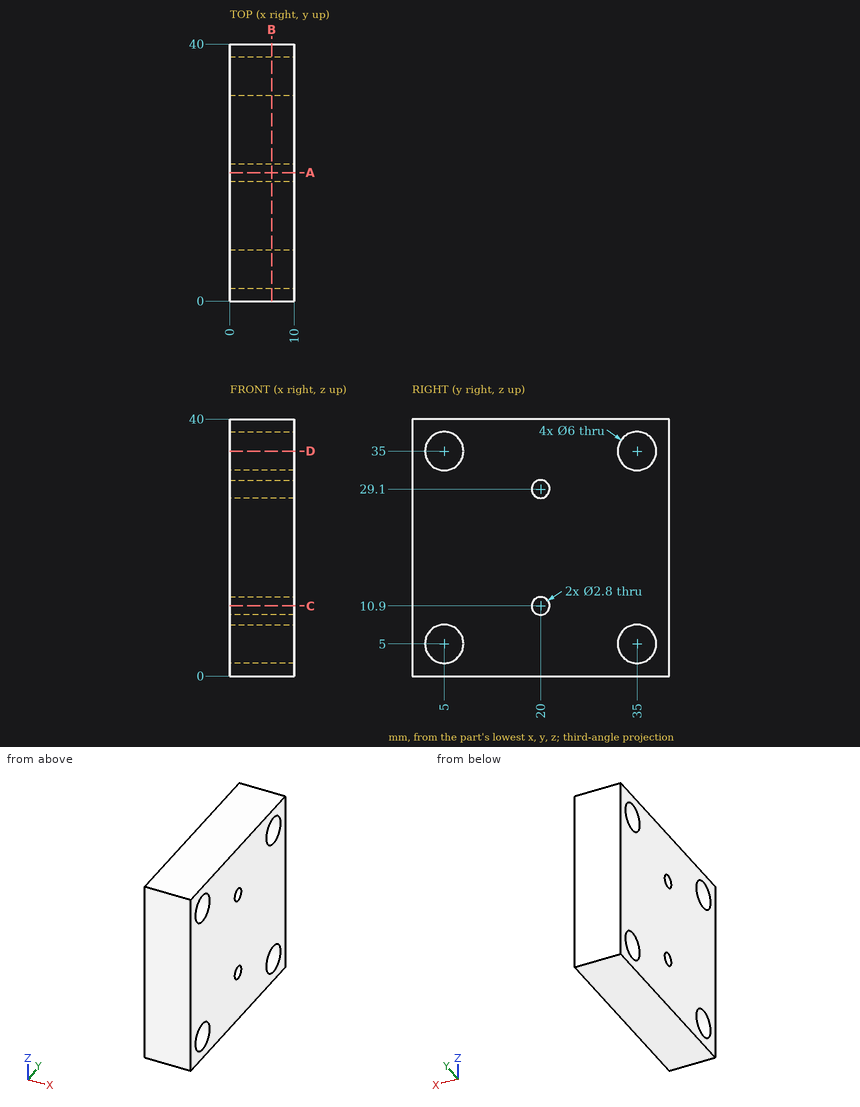
Could you check a few things on this drawing? It's one solid part, dimensions in mm from its lowest x, y, z. Coordinates: 2 decimals unless noted, no trailing zeros. Order: outer loops, then holes, each group sorted by start corner. A loop starts at its lowest first (then second) coordinate and runs counter-clockwise, first axis right, second up.
1. If we section it at A-A (y = 20): Please give me the cut outline in (x, z), then the cut area to 3 significant figures.
2. If we section it at D-D (z = 35): Please give me the cut outline in (x, y).
3. I'm going to push a flat-ended pin straight in: pin 1 (2 mm diameter, centred on y = 20, z = 29.1, fed in from +X). Where does the tip first touch, or does it pass through?
4. I need wall thicknesses on line 1 (Y direction, x = 3.25, z = 5); line 2 (Z direction, x = 4.5, y = 33); line 3 (Y direction, x = 5, z = 29). Which ranges of each line are inside material? Lowest first, please.
5. If we section it at C-C (z = 10.9): Please give me the cut outline in (x, y).
6. If we section it at B-B (x = 6.5): Please give me the cut outline in (y, z), then the cut area to 3 significant figures.
Entries:
1. outline: (0, 0) - (10, 0) - (10, 9.5) - (0, 9.5) - close; (0, 12.3) - (10, 12.3) - (10, 27.7) - (0, 27.7) - close; (0, 30.5) - (10, 30.5) - (10, 40) - (0, 40) - close
1. area: 344 mm2
2. outline: (0, 0) - (10, 0) - (10, 2) - (0, 2) - close; (0, 8) - (10, 8) - (10, 32) - (0, 32) - close; (0, 38) - (10, 38) - (10, 40) - (0, 40) - close
3. pin 1: passes through
4. line 1: y = 0 to 2, 8 to 32, 38 to 40
4. line 2: z = 0 to 2.76, 7.24 to 32.76, 37.24 to 40
4. line 3: y = 0 to 18.6, 21.4 to 40
5. outline: (0, 0) - (10, 0) - (10, 18.6) - (0, 18.6) - close; (0, 21.4) - (10, 21.4) - (10, 40) - (0, 40) - close
6. outline: (0, 0) - (40, 0) - (40, 40) - (0, 40) - close; hole circle Ø6 at (5, 5); hole circle Ø6 at (5, 35); hole circle Ø2.8 at (20, 10.9); hole circle Ø2.8 at (20, 29.1); hole circle Ø6 at (35, 5); hole circle Ø6 at (35, 35)
6. area: 1,470 mm2
